```python
from build123d import *

# Parameters (mm, degrees)
SKETCH1_W               = 17.78
SKETCH1_H               = 2.54
BOSS_EXTRUDE1_DEPTH     = 11.43
SKETCH2_W               = 17.78
SKETCH2_H               = 2.54
BOSS_EXTRUDE2_DEPTH     = 15.24
SKETCH16_W              = 3.81
SKETCH16_H              = 2.54
BOSS_EXTRUDE10_DEPTH    = 7.62
BOSS_EXTRUDE11_REACH    = 36.757
SKETCH17_W              = 5.08
SKETCH17_H              = 2.54
MIRROR3_COPY_1_SKETCH_W = 3.81
MIRROR3_COPY_1_SKETCH_H = 2.54
MIRROR3_COPY_1_DEPTH    = 7.62
MIRROR3_COPY_2_REACH    = 36.757
MIRROR3_COPY_2_SKETCH_W = 5.08
MIRROR3_COPY_2_SKETCH_H = 2.54
SKETCH18_W              = 5.08
SKETCH18_H              = 17.78
BOSS_EXTRUDE12_DEPTH    = 5.08
SKETCH19_W              = 17.78
SKETCH19_H              = 2.54
BOSS_EXTRUDE13_DEPTH    = 5.08
FILLET1_R               = 2.54


with BuildPart() as part:
    # Sketch1 → Boss-Extrude1 (new body)
    with BuildSketch(Plane(origin=(0, 0, 0), x_dir=(0, 0, -1), z_dir=(1, 0, 0))):
        with Locations((0, 1.27)):
            Rectangle(SKETCH1_W, SKETCH1_H)
    extrude(amount=BOSS_EXTRUDE1_DEPTH)

    # Sketch2 → Boss-Extrude2 (add)
    with BuildSketch(Plane.ZY):
        with Locations((0, 1.27)):
            Rectangle(SKETCH2_W, SKETCH2_H)
    extrude(amount=BOSS_EXTRUDE2_DEPTH)

    # Mirror1: part across plane


with BuildPart() as part_1:
    add(part.part)
    add(part.part.mirror(Plane.ZY.offset(15.24)))

    # Sketch16 → Boss-Extrude10 (add)
    with BuildSketch(Plane.XY.offset(8.89)):
        with Locations((-17.145, 1.27)):
            Rectangle(SKETCH16_W, SKETCH16_H)
        with Locations((-40.005, 1.27)):
            Rectangle(SKETCH16_W, SKETCH16_H)
    boss_extrude10 = extrude(amount=BOSS_EXTRUDE10_DEPTH)

    # Sketch17 → Boss-Extrude11 (add, up to next)
    with BuildSketch(Plane.ZY.offset(19.05), mode=Mode.PRIVATE) as boss_extrude11_sk1:
        with Locations((13.97, 1.27)):
            Rectangle(SKETCH17_W, SKETCH17_H)
    boss_extrude11_tool1 = extrude(boss_extrude11_sk1.sketch, amount=BOSS_EXTRUDE11_REACH, mode=Mode.PRIVATE) - part_1.part
    boss_extrude11 = boss_extrude11_tool1.solids().sort_by_distance((-19.05, 1.27, 13.97))[0]
    add(boss_extrude11)

    # Mirror2: Boss-Extrude10, Boss-Extrude11 across plane
    add(boss_extrude10.mirror(Plane.ZY.offset(15.24)))
    add(boss_extrude11.mirror(Plane.ZY.offset(15.24)))

    # Mirror3: Boss-Extrude10, Boss-Extrude11 across plane
    add(boss_extrude10.mirror(Plane.XY))
    add(boss_extrude11.mirror(Plane.XY))

    # Mirror3 copy 1 sketch → Mirror3 copy 1 (add)
    with BuildSketch(Plane(origin=(-30.48, 0, -8.89), x_dir=(-1, 0, 0), z_dir=(0, 0, -1))):
        with Locations((-17.145, 1.27)):
            Rectangle(MIRROR3_COPY_1_SKETCH_W, MIRROR3_COPY_1_SKETCH_H)
        with Locations((-40.005, 1.27)):
            Rectangle(MIRROR3_COPY_1_SKETCH_W, MIRROR3_COPY_1_SKETCH_H)
    extrude(amount=MIRROR3_COPY_1_DEPTH)

    # Mirror3 copy 2 sketch → Mirror3 copy 2 (add, up to next)
    with BuildSketch(Plane(origin=(-11.43, 0, 0), x_dir=(0, 0, -1), z_dir=(1, 0, 0)), mode=Mode.PRIVATE) as mirror3_copy_2_sk1:
        with Locations((13.97, 1.27)):
            Rectangle(MIRROR3_COPY_2_SKETCH_W, MIRROR3_COPY_2_SKETCH_H)
    mirror3_copy_2_tool1 = extrude(mirror3_copy_2_sk1.sketch, amount=MIRROR3_COPY_2_REACH, mode=Mode.PRIVATE) - part_1.part
    add(mirror3_copy_2_tool1.solids().sort_by_distance((-11.43, 1.27, -13.97))[0])

    # Sketch18 → Boss-Extrude12 (add)
    with BuildSketch(Plane.XZ):
        with Locations((-2.54, 0)):
            Rectangle(SKETCH18_W, SKETCH18_H)
    boss_extrude12 = extrude(amount=BOSS_EXTRUDE12_DEPTH)

    # Sketch19 → Boss-Extrude13 (add)
    with BuildSketch(Plane.ZY.offset(5.08)):
        with Locations((0, -3.81)):
            Rectangle(SKETCH19_W, SKETCH19_H)
    boss_extrude13 = extrude(amount=BOSS_EXTRUDE13_DEPTH)

    # Mirror4: Boss-Extrude12, Boss-Extrude13 across plane
    add(boss_extrude12.mirror(Plane.ZY.offset(15.24)))
    add(boss_extrude13.mirror(Plane.ZY.offset(15.24)))

    # Fillet1
    fillet1_edges = [part_1.edges().sort_by_distance(p)[0] for p in [
        (-41.91, 1.27, -16.51),
        (11.43, 1.27, -16.51),
        (-41.91, 1.27, 16.51),
        (11.43, 1.27, 16.51),
    ]]
    fillet(fillet1_edges, radius=FILLET1_R)


solid = part_1.part
```
Model file for the job. Use its own axes, mm. A direction names the side the tool comes from. Round coordinates to 2 decimals unless told otherwise and drop trailing zeros. Write each loop counter-clockwise with the first axis right and the second up, starting at its lowest first coordinate (ties: lowest second). Pieces come first, ordered by that corner, then holes. Notation, with made-up numbers: (-10.75, 23) -> (1.25, 23) arc R20 cw to (1.25, 56) -> close; hole circle Ø4 at (35, 32.25). An arc over 180 degrees is marked (long way). Answer as CSV lines item,"result".
1. Pin check, flat tips, straight feed: pin 1 Ø2.5 at (x, y) = (-31.5, -2) entering from +Z; pin 2 Ø1 at (x, z) = (-17, -3.5) entering from -Y; pin 3 Ø3 at (y, z) = (-4, -3) entering from -X. Stop position of each tip, or through.
Resolved:
pin 1,"z = 8.89"
pin 2,"y = 0"
pin 3,"x = -30.48"
2. Slice it at D-D, the plane y = -4.5. List the corners of the cut face in (x, z), plus the area to 3 significant figures.
Resolved:
outline,"(-30.48, -8.89) -> (-20.32, -8.89) -> (-20.32, 8.89) -> (-30.48, 8.89) -> close; (-10.16, -8.89) -> (0, -8.89) -> (0, 8.89) -> (-10.16, 8.89) -> close"
area,"361 mm²"
3. Slice it at B-B, the plane y = 1.5. List the corners of the cut face in (x, z).
Resolved:
outline,"(-41.91, -13.97) arc R2.54 ccw to (-39.37, -16.51) -> (8.89, -16.51) arc R2.54 ccw to (11.43, -13.97) -> (11.43, 13.97) arc R2.54 ccw to (8.89, 16.51) -> (-39.37, 16.51) arc R2.54 ccw to (-41.91, 13.97) -> close; hole (-38.1, -11.43) -> (-19.05, -11.43) -> (-19.05, -8.89) -> (-38.1, -8.89) -> close; hole (-38.1, 8.89) -> (-19.05, 8.89) -> (-19.05, 11.43) -> (-38.1, 11.43) -> close; hole (-11.43, -11.43) -> (7.62, -11.43) -> (7.62, -8.89) -> (-11.43, -8.89) -> close; hole (-11.43, 8.89) -> (7.62, 8.89) -> (7.62, 11.43) -> (-11.43, 11.43) -> close"
4. Slice it at A-A, the plane x = -35.5. List the corners of the cut face in (y, z), plus the area to 3 significant figures.
Resolved:
outline,"(0, -16.51) -> (2.54, -16.51) -> (2.54, -11.43) -> (0, -11.43) -> close; (0, -8.89) -> (2.54, -8.89) -> (2.54, 8.89) -> (0, 8.89) -> close; (0, 11.43) -> (2.54, 11.43) -> (2.54, 16.51) -> (0, 16.51) -> close"
area,"71.0 mm²"
5. Mould opens along X. For faces 5 (the face through (-16, 1, -16.51)), 6 (the face through (-2, 0, 8.89)), 7 (the face through (10.706, 1.288, 15.746)) say: +X half, -X half, draft (parallel to the pull), parting line (faces both ways), or undercut.
Resolved:
face 5,"draft"
face 6,"undercut"
face 7,"+X half"
6. Slice it at C-C, the plane x = -24.5. List the corners of the cut face in (y, z).
Resolved:
outline,"(-5.08, -8.89) -> (-2.54, -8.89) -> (-2.54, 8.89) -> (-5.08, 8.89) -> close; (0, -16.51) -> (2.54, -16.51) -> (2.54, -11.43) -> (0, -11.43) -> close; (0, -8.89) -> (2.54, -8.89) -> (2.54, 8.89) -> (0, 8.89) -> close; (0, 11.43) -> (2.54, 11.43) -> (2.54, 16.51) -> (0, 16.51) -> close"
7. Drill centre lines: line 1 (Z direction, x = -31, y = 1.5); line 2 (X direction, y = -4, z = 8); line 3 (Y direction, x = 6.5, z = 8.5). Where is each one in solid material? Low to high.
Resolved:
line 1,"-16.51 to -11.43, -8.89 to 8.89, 11.43 to 16.51"
line 2,"-30.48 to -20.32, -10.16 to 0"
line 3,"0 to 2.54"
8. Tool access for faces 1 (the face through (-2, 1, -11.43)), 2 (the face through (-30.48, -3, 0)), 3 (the face through (-8, -2.54, 0)), 4 (the face through (-10.16, -4, 0)): list every direction of +Z, -Z, +X, -X, +Y, -Y with a clear straight run to the whole face (end or side of a thin tool).
Resolved:
face 1,"+Y, -Y"
face 2,"+Z, -Z, -X, -Y"
face 3,"+Z, -Z"
face 4,"+Z, -Z, -Y"
